Study the drawing (mm; zero at the part's minimum x, y, z) and answer. Coordinates: 2 decimals unless noted, no trailing zeros. Order: outer loops, then holes, each group sorted by start corner. A loop starts at its lowest first (then second) coordinate and runs counter-clockwise, first axis right, second up.
1. Determine the mould class of the marked faces 1, 2 and 3 for opening direction Y: +Y half, -Y half, draft (parallel to the pull), parting line (faces both ways), or undercut.
2. Find the intervals of material crossed by probe 1 along Z at (x, y) = (40, 10); probe 2 along Y at (x, z) = (40, 44); probe 3 along Y at (x, z) = (46, 37), in increasing order.
3. Flat-ended cylindrical pins translate along their axes: pin 1 Ø4 at (x, z) = (59.5, 27.5) entering from -Y; pin 2 Ø12 at (x, z) = (23, 92.5) entering from +Y; pin 3 Ø10 at (x, z) = (13.5, 67.5) entering from -Y; pin 4 Ø24.5 at (x, y) = (40, 40) entering from +Z. Find the tip coordinate at first contact, or state that the pin passes through.
4. The part is cut by section D-D, the plane y = 16. Give the vertices of the cut face in (x, z).
5. The part is cut by section B-B, the plane y = 40. Give the vertices of the cut face in (x, z).
6. The part is cut by section C-C, the plane z = 81. Give the vertices of the cut face in (x, y), then the cut area to 3 significant figures.
7. The part is cut by section A-A, the plane x = 40. Give the vertices of the cut face in (y, z), then the cut area to 3 significant figures.
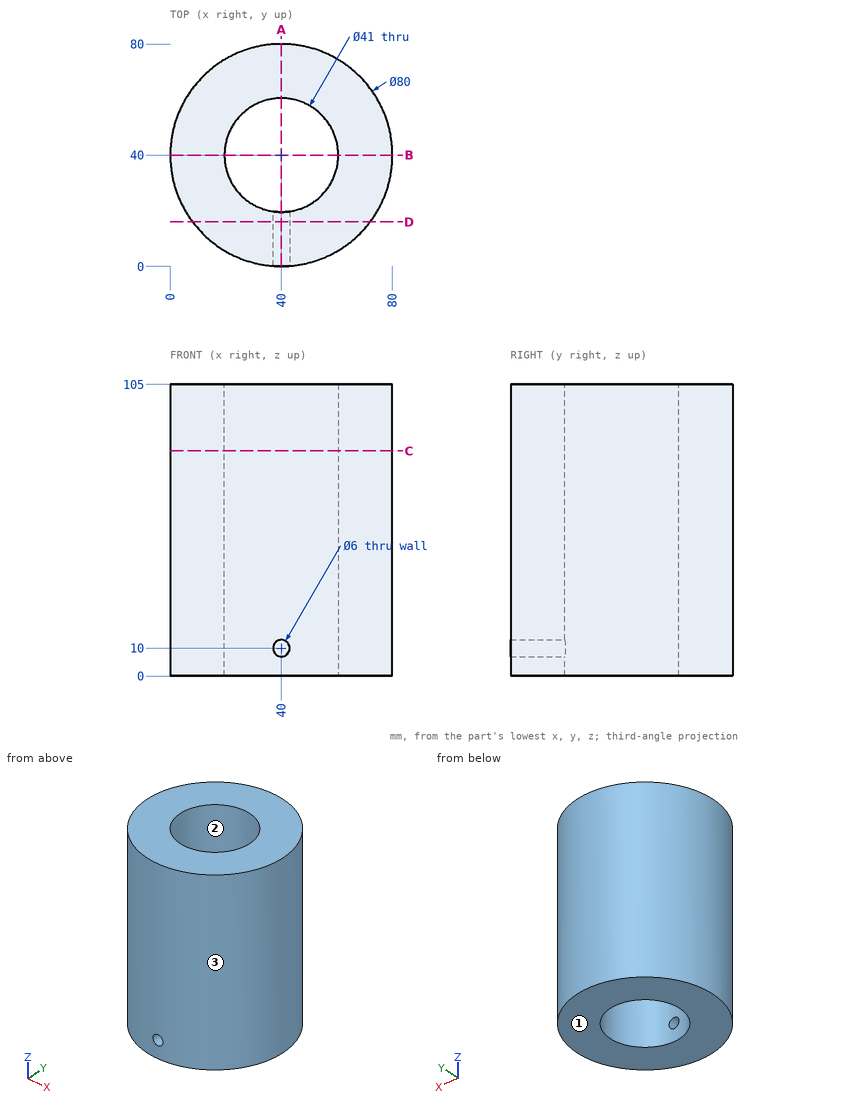
Geometry says:
1. face 1: draft
1. face 2: undercut
1. face 3: parting line
2. probe 1: z = 0 to 7, 13 to 105
2. probe 2: y = 0 to 19.5, 60.5 to 80
2. probe 3: y = 0.45 to 20.4, 59.6 to 79.55
3. pin 1: stops at y = 4.03
3. pin 2: stops at y = 78.46
3. pin 3: stops at y = 6.27
3. pin 4: passes through
4. outline: (8, 0) - (72, 0) - (72, 105) - (8, 105) - close; hole circle Ø6 at (40, 10)
5. outline: (0, 0) - (19.5, 0) - (19.5, 105) - (0, 105) - close; (60.5, 0) - (80, 0) - (80, 105) - (60.5, 105) - close
6. outline: circle Ø80 at (40, 40); hole circle Ø41 at (40, 40)
6. area: 3,710 mm2
7. outline: (0, 0) - (19.5, 0) - (19.5, 7) - (0, 7) - close; (0, 13) - (19.5, 13) - (19.5, 105) - (0, 105) - close; (60.5, 0) - (80, 0) - (80, 105) - (60.5, 105) - close
7. area: 3,980 mm2
